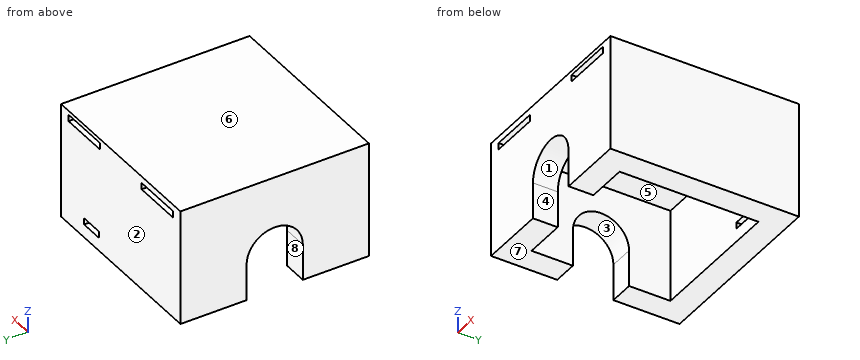
```python
from build123d import *

# Parameters (mm, degrees)
SKETCH2_W           = 57
SKETCH2_H           = 57
BOSS_EXTRUDE1_DEPTH = 35
SKETCH3_W           = 15
SKETCH3_H           = 2
CUT_EXTRUDE1_DEPTH  = 60
SKETCH4_W           = 42
SKETCH4_H           = 42
CUT_EXTRUDE2_DEPTH  = 28
CUT_EXTRUDE4_DEPTH  = 5
CUT_EXTRUDE5_DEPTH  = 10
CUT_EXTRUDE6_DEPTH  = 5
SKETCH13_W          = 7
SKETCH13_H          = 1.952566844
CUT_EXTRUDE8_DEPTH  = 12


with BuildPart() as part:
    # Sketch2 → Boss-Extrude1 (new body)
    with BuildSketch(Plane.XY):
        with Locations((-5.733009709, -0.737864078)):
            Rectangle(SKETCH2_W, SKETCH2_H)
    extrude(amount=BOSS_EXTRUDE1_DEPTH)

    # Sketch3 → Cut-Extrude1 (cut)
    with BuildSketch(Plane(origin=(0, 27.762135922, 0), x_dir=(1, 0, 0), z_dir=(0, 1, 0))):
        with Locations((-23.156416284, -32)):
            Rectangle(SKETCH3_W, SKETCH3_H)
        with Locations((11.686990291, -32.761209032)):
            Rectangle(SKETCH3_W, SKETCH3_H)
    extrude(amount=-CUT_EXTRUDE1_DEPTH, mode=Mode.SUBTRACT)

    # Sketch4 → Cut-Extrude2 (cut)
    with BuildSketch(Plane(origin=(0, 0, 0), x_dir=(-1, 0, 0), z_dir=(0, 0, -1))):
        with Locations((5.733009709, -0.737864078)):
            Rectangle(SKETCH4_W, SKETCH4_H)
    extrude(amount=-CUT_EXTRUDE2_DEPTH, mode=Mode.SUBTRACT)

    # Sketch5 → Cut-Extrude4 (cut)
    with BuildSketch(Plane(origin=(0, -21.737864078, 0), x_dir=(1, 0, 0), z_dir=(0, 1, 0))):
        with BuildLine():
            Line((2.766990291, -11), (2.766990291, 0))
            Line((2.766990291, 0), (-14.233009709, 0))
            Line((-14.233009709, 0), (-14.233009709, -11))
            ThreePointArc((-14.233009709, -11), (-5.733009709, -19.5), (2.766990291, -11))
        make_face()
    extrude(amount=-CUT_EXTRUDE4_DEPTH, mode=Mode.SUBTRACT)

    # Sketch7 → Cut-Extrude5 (cut)
    with BuildSketch(Plane(origin=(-26.733009709, 0, 0), x_dir=(0, 0, -1), z_dir=(1, 0, 0))):
        with BuildLine():
            Line((-11, -9.237864078), (0, -9.237864078))
            Line((0, -9.237864078), (0, 7.762135922))
            Line((0, 7.762135922), (-11, 7.762135922))
            ThreePointArc((-11, 7.762135922), (-19.5, -0.737864078), (-11, -9.237864078))
        make_face()
    extrude(amount=-CUT_EXTRUDE5_DEPTH, mode=Mode.SUBTRACT)

    # Sketch8 → Cut-Extrude6 (cut)
    with BuildSketch(Plane(origin=(0, -26.737864078, 0), x_dir=(1, 0, 0), z_dir=(0, 1, 0))):
        with BuildLine():
            Line((-14.233009709, 0), (2.766990291, 0))
            Line((2.766990291, 0), (2.766990291, -11))
            ThreePointArc((2.766990291, -11), (-5.733009709, -19.5), (-14.233009709, -11))
            Line((-14.233009709, -11), (-14.233009709, 0))
        make_face()
    extrude(amount=-CUT_EXTRUDE6_DEPTH, mode=Mode.SUBTRACT)

    # Sketch13 → Cut-Extrude8 (cut)
    with BuildSketch(Plane(origin=(0, 27.762135922, 0), x_dir=(1, 0, 0), z_dir=(0, 1, 0))):
        with Locations((8.266990291, -4.976283422)):
            Rectangle(SKETCH13_W, SKETCH13_H)
    extrude(amount=-CUT_EXTRUDE8_DEPTH, mode=Mode.SUBTRACT)


solid = part.part
```
Can you work these out from the model? Positions are in its coordinate system, mm. Face numbers are marked on the shaded views. A direction names the side the tool comes from. Give positions to 0.01 mm unless a question says otherwise; leave off trailing zeros. Order: outer loops, then holes, each group sorted by start corner. A loop starts at its lowest first (then second) coordinate and runs counter-clockwise, first axis right, second up. Notation, with made-up numbers: M 33.5,33 L 47.5,33 A16 ccw 47.5,60 Z; hole C -32.75,56.25 d3. An arc over 180 degrees is marked long. Write item = value, one per line. Start each with the question number.
Q1. Suppose I cut it at A-A (x = -26). Write out the boundary of the cut face in (y, z), plus the area to 3 significant figures.
Q2. Suppose I cut it at C-C (y = 23). Write out the boundary of the cut face in (x, z), plus the area to 3 significant figures.
Q3. Will these pins go through, and if not, where does the flat tip stop? pin 1 Ø4.5 at (x, y) = (12.5, -2.5) entering from -Z; pin 2 Ø3 at (x, z) = (-11, 4.5) entering from -Y.
Q4. I need wall thicknesses on probe 1 along Y at (x, z) = (-3, 24); probe 2 along Y at (x, z) = (-27, 4.5); probe 3 along X at (y, z) = (16, 25). Which ranges of each line are inside material? Lowest first, please. Write a range as [from, to].
Q5. Suppose I cut it at D-D (y = -6). Write out the boundary of the cut face in (x, z), plus the area to 3 significant figures.
Q6. For the marked faces 4, 5, 6, 7 and 8, which set-ups out of +Z, -Z, +X, -X, +Y, -Y let a thin tool reach every point of the face, with its end or its side?
Q7. Suppose I cut it at B-B (z = 2.5). Write out the boundary of the cut face in (x, y).
Q8. We'd pull the mould along Y, two halves only. Please class the marked faces 1, 2 and 3: pulls with the +Y half, pulls with the -Y half, needs draft (parallel to the pull), parting line crosses it, or undercut.
Check result:
q1.outline = M -29.24,0 L -21.74,0 L -21.74,28 L 20.26,28 L 20.26,0 L 27.76,0 L 27.76,31 L -29.24,31 Z; M -29.24,33 L 27.76,33 L 27.76,35 L -29.24,35 Z
q1.area = 705 mm2
q2.outline = M -34.23,0 L 22.77,0 L 22.77,35 L -34.23,35 Z; hole M -30.66,31 L -15.66,31 L -15.66,33 L -30.66,33 Z; hole M 4.19,31.76 L 19.19,31.76 L 19.19,33.76 L 4.19,33.76 Z; hole M 4.77,4 L 11.77,4 L 11.77,5.95 L 4.77,5.95 Z
q2.area = 1,920 mm2
q3.pin_1 = 28
q3.pin_2 = 20.26
q4.probe_1 = [-29.24, -21.74], [20.26, 27.76]
q4.probe_2 = [-29.24, -9.24], [7.76, 27.76]
q4.probe_3 = [-34.23, -26.73], [15.27, 22.77]
q5.outline = M -34.23,17.68 L -26.73,17.68 L -26.73,28 L 15.27,28 L 15.27,0 L 22.77,0 L 22.77,35 L -34.23,35 Z; hole M -30.66,31 L -15.66,31 L -15.66,33 L -30.66,33 Z; hole M 4.19,31.76 L 19.19,31.76 L 19.19,33.76 L 4.19,33.76 Z
q5.area = 626 mm2
q6.face_4 = -Z, -Y
q6.face_5 = -Z
q6.face_6 = +Z, +X, -X, +Y, -Y
q6.face_7 = -Z, +X, -X, +Y, -Y
q6.face_8 = -Z, -X
q7.outline = M -34.23,-29.24 L -14.23,-29.24 L -14.23,-21.74 L -26.73,-21.74 L -26.73,-9.24 L -34.23,-9.24 Z; M -34.23,7.76 L -26.73,7.76 L -26.73,20.26 L 15.27,20.26 L 15.27,-21.74 L 2.77,-21.74 L 2.77,-29.24 L 22.77,-29.24 L 22.77,27.76 L -34.23,27.76 Z
q8.face_1 = needs draft
q8.face_2 = pulls with the +Y half
q8.face_3 = undercut
